The drawing under review shows one solid part. Ordinate dimensions are in mm from its lowest x, y, z. A direction names the side the tool comes from. Round coordinates to 2 decimals unless told otherwise and drop trailing zeros. Loops run counter-clockwise (first coordinate to the right, second up) from the corner with the lowest first, then second, coordinate; pieces in that order, holes last. Notation, with made-up numbers: M -30,43.5 L 9,43.5 A28 ccw 9,63.5 Z; hole C 38.5,-6 d7. An arc over 180 degrees is marked long. Use a Markdown table: item, result.
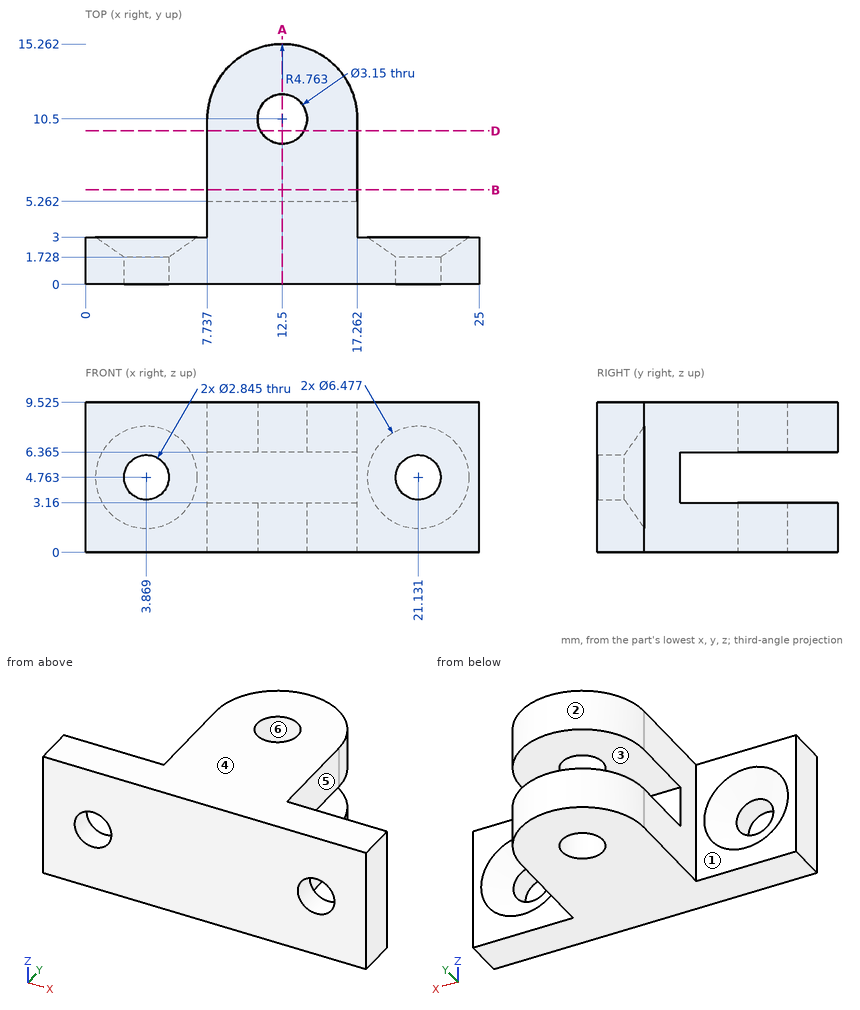
1. Wall thickness on line 1 along X through (y, z) = (10.5, 7.1) (1 decimal); line 2 along Z through (x, y) = (9, 8.75) (1 decimal); line 3 along Y through (x, z) = (12.5, 1.25) (1 decimal): over which ranges is each line inside the solid? List them lowest first. Write a range as from..to.
Check values:
| item | result |
|---|---|
| line 1 | x = 7.7..10.9, 14.1..17.3 |
| line 2 | z = 0..3.2, 6.4..9.5 |
| line 3 | y = 0..8.9, 12.1..15.3 |
2. Insertion check: pin 1 (1 mm diameter, centred on x = 13, z = 4, fed in from +Y); pin 2 (2 mm diameter, centred on x = 10.5, z = 5.5, fed in from -Y); pin 3 (5 mm diameter, centred on y = 11, z = 2, fed in from -X); pin 4 (5 mm diameter, centred on x = 9, z = 3.5, fed in from +Y). Each pin has a flat end and moves straight along its axis. Give the tip position at first contact, or say it passes through.
Check values:
| item | result |
|---|---|
| pin 1 | stops at y = 5.26 |
| pin 2 | stops at y = 0 |
| pin 3 | stops at x = 7.74 |
| pin 4 | stops at y = 15.15 |
3. Take a section at A-A on x = 12.5. Give the boundary of the cut face in (y, z) (1 decimal).
Check values:
| item | result |
|---|---|
| outline | M 0,0 L 8.9,0 L 8.9,3.2 L 5.3,3.2 L 5.3,6.4 L 8.9,6.4 L 8.9,9.5 L 0,9.5 Z; M 12.1,0 L 15.3,0 L 15.3,3.2 L 12.1,3.2 Z; M 12.1,6.4 L 15.3,6.4 L 15.3,9.5 L 12.1,9.5 Z |
4. The part is to be moulded in two halves that separate along X. For the marked faces 4, 5 and 6, say which applies: pulls with the +X half, pulls with the -X half, needs draft (parallel to the pull), parting line crosses it, or undercut.
Check values:
| item | result |
|---|---|
| face 4 | needs draft |
| face 5 | pulls with the +X half |
| face 6 | undercut |
5. Take a section at B-B on y = 6. Give the boundary of the cut face in (x, z) (1 decimal).
Check values:
| item | result |
|---|---|
| outline | M 7.7,0 L 17.3,0 L 17.3,3.2 L 7.7,3.2 Z; M 7.7,6.4 L 17.3,6.4 L 17.3,9.5 L 7.7,9.5 Z |
6. Take a section at D-D on y = 9.75. Give the boundary of the cut face in (x, z) (1 decimal).
Check values:
| item | result |
|---|---|
| outline | M 7.7,0 L 11.1,0 L 11.1,3.2 L 7.7,3.2 Z; M 7.7,6.4 L 11.1,6.4 L 11.1,9.5 L 7.7,9.5 Z; M 13.9,0 L 17.3,0 L 17.3,3.2 L 13.9,3.2 Z; M 13.9,6.4 L 17.3,6.4 L 17.3,9.5 L 13.9,9.5 Z |
7. Machinability: for the marked faces 1, 2 and 3, which of the approach directions +Z, -Z, +X, -X, +Y, -Y give a long, thin tool a straight path to every point of the face, cutting with its end or side? Answer none if there is none.
Check values:
| item | result |
|---|---|
| face 1 | +Z, -Z, -X, +Y |
| face 2 | +Z, -Z, +Y |
| face 3 | +X, -X, +Y |
